```python
from build123d import *

# Parameters (mm, degrees)
F0_W     = 38.1
F0_H     = 60.325
F1_DEPTH = 34.925
F3_DEPTH = 25.4
F5_DEPTH = 25.4
F6_W     = 25.0000946254
F6_H     = 12.7
F7_DEPTH = 25.4


with BuildPart() as f1:
    # F0 (on Front) → F1 (new body)
    with BuildSketch(Plane.XZ):
        with Locations((19.05, 30.1625)):
            Rectangle(F0_W, F0_H)
    extrude(amount=F1_DEPTH)

    # F2 (on face) → F3 (join)
    with BuildSketch(Plane.YZ.offset(38.1)):
        Polygon((-9.9249053746, 60.325), (-34.925, 12.7), (-9.9249053746, 12.7), align=None)
    extrude(amount=F3_DEPTH)

    # F4 (on face) → F5 (join)
    with BuildSketch(Plane.YZ.offset(38.1)):
        Polygon((0, 60.325), (-9.9249053746, 60.325), (-9.9249053746, 12.7), (-9.9249053746, 0), (0, 0), align=None)
    extrude(amount=F5_DEPTH)

    # F6 (on face) → F7 (join)
    with BuildSketch(Plane.YZ.offset(38.1)):
        with Locations((-22.4249526873, 6.35)):
            Rectangle(F6_W, F6_H)
    extrude(amount=F7_DEPTH)


solid = f1.part
```
Check sheet for the modelled part. Datum: model origin and axes. Units: mm. A direction names the side the tool comes from. Coordinates: 2 decimals unless noted, no trailing zeros. Loops run counter-clockwise (first coordinate to the right, second up) from the corner with the lowest first, then second, coordinate; pieces in that order, holes last. Notation, with made-up numbers: M 78,-28.75 L 106,-28.75 A23 cw 106,-19.75 Z; hole C -1.5,76 d4. An arc over 180 degrees is marked long. Answer as a JSON object with one key per item and string values.
1. Sectioned sample at B-B on z = 31. Record the cut outline in (x, y) (3 decimals), and give its area (3 significant figures).
Outcome:
{"outline": "M 0,-34.925 L 38.1,-34.925 L 38.1,-25.319 L 63.5,-25.319 L 63.5,0 L 0,0 Z", "area": "1,970 mm²"}
2. Sectioned sample at C-C on y = -20.5. Record the cut outline in (x, z) (3 decimals), and give its area (3 significant figures).
Outcome:
{"outline": "M 0,0 L 63.5,0 L 63.5,40.18 L 38.1,40.18 L 38.1,60.325 L 0,60.325 Z", "area": "3,320 mm²"}
3. Sectioned sample at A-A on x = 56.5. Record the cut outline in (y, z) (3 decimals).
Outcome:
{"outline": "M -34.925,0 L 0,0 L 0,60.325 L -9.925,60.325 L -34.925,12.7 Z"}
4. Scan lines: L1, parallel to X at y = -33, z = 32.5; L2, parallel to Y at x = 52.5, z = 26; L3, parallel to Y at x = 60, z = 30. Record each from-to range of solid material in increasing order. Write a range as from..to.
Outcome:
{"L1": "0..38.1", "L2": "-27.94..0", "L3": "-25.84..0"}
5. Depth check by flat-ended pin: P1, Ø2, axis at y = -19.5, z = 51, coming from the -X side; P2, Ø4, axis at x = 55, z = 26, coming from the -Y side; P3, Ø12, axis at x = 56, z = 32, coming from the -Y side. Enter the tip coordinate at first touch or a pass-through.
Outcome:
{"P1": "x = 0", "P2": "y = -28.99", "P3": "y = -27.94"}
6. Access from +Z, -Z, +X, -X, +Y, -Y to the whole of each face (thin tool, end or side, straight path). Record for faces 1 (the flat face through (50.62, -22.25, 36.85)), 2 (the flat face through (0, -17, 30)).
Outcome:
{"face 1": "+Z, +X, -Y", "face 2": "+Z, -Z, -X, +Y, -Y"}
